Source: CAD feature listing. Evaluate the final solid. Frame: model axes, mm. Face numbers are marked on the shaded views. A direction names the side the tool comes from. Give positions to 0.01 mm unless a question says otherwise; leave off trailing zeros. Order: outer loops, then holes, each group sorted by start corner. A loop starts at its lowest first (then second) coordinate and runs counter-clockwise, first axis right, second up.
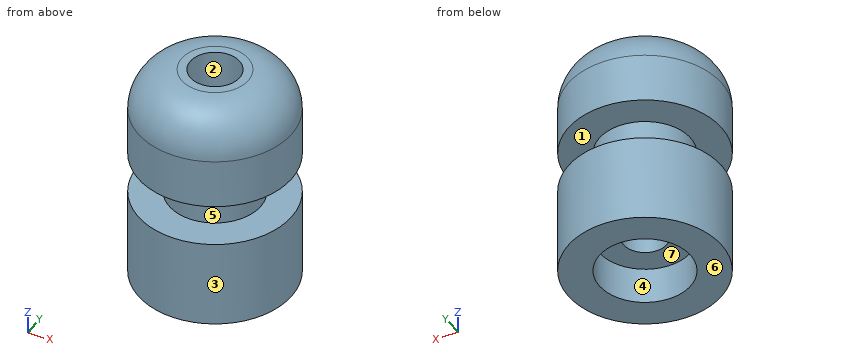
from build123d import *

# Parameters (mm, degrees)
F3_D = 10
F4_R = 10


with BuildPart() as f1:
    # F0 (on Front) → F1 (revolve)
    with BuildSketch(Plane.XZ):
        Polygon((7.1379574947, 42.9636351764), (-4.8425933346, 42.9636351764), (-4.8425933346, 27.8560947627), (-10.5409119278, 27.8560947627), (-10.5409119278, 0), (0, 0), (0, -8.4736431018), (7.1379574947, -8.4736431018), (7.1379574947, 11.8357595056), (0, 11.8357595056), (0, 21.5210486203), (7.1379574947, 21.5210486203), align=None)
    revolve(axis=Axis((-10.5409119278, 0, 16.1306988448), (0, 0, -1)))

    # F3 (through all)
    with Locations(Plane(origin=(0, 0, 0), x_dir=(1, 0, 0), z_dir=(0, 0, -1))):
        with Locations((-10.5409119278, 0)):
            Hole(F3_D / 2)

    # F4
    f4_edges = [f1.edges().sort_by_distance(p)[0] for p in [
        (-28.219781, 0, 42.963635),
    ]]
    fillet(f4_edges, radius=F4_R)


solid = f1.part
1) Section query A-A on z = -3. Output: boundary loops of the cut face in (x, y), and give its area (3 significant figures).
Checks:
outline: circle Ø35.36 at (-10.54, 0); hole circle Ø21.08 at (-10.54, 0)
area: 633 mm2
2) Ray query, L1, parallel to X at y = 0, z = -3.5; L2, parallel to Z at x = -15, y = -11; L3, parallel to Z at x = 5, y = -4. Return the intervals inside material, ascending.
Checks:
L1: x = -28.22 to -21.08, 0 to 7.14
L2: z = -8.47 to 11.84, 21.52 to 42.04
L3: z = -8.47 to 11.84, 21.52 to 38.44
3) Section query B-B on z = 10.5. Output: boundary loops of the cut face in (x, y).
Checks:
outline: circle Ø35.36 at (-10.54, 0); hole circle Ø10 at (-10.54, 0)
4) Pull-direction query (X, two-part tool) for the marked faces 4, 5, 6 and 7; classes: +X half, -X half, draft (parallel to the pull), parting line (faces both ways), or undercut.
Checks:
face 4: undercut
face 5: parting line
face 6: draft
face 7: undercut
5) First-contact query: pin 1 Ø3 at (x, z) = (-15.5, 13) entering from +Y; pin 2 Ø4 at (x, z) = (-14.5, 9.5) entering from +Y; pin 3 Ø10 at (x, y) = (-7.5, -4) entering from +Z; pin 4 Ø1.5 at (x, y) = (-17, 6) entering from -Z. Flat tips, straight axial feed; report the tip coordinate or a pass-through.
Checks:
pin 1: stops at y = 17.22
pin 2: stops at y = 17.57
pin 3: stops at z = 42.96
pin 4: stops at z = 0
6) Reachability of the marked faces 1, 2 and 3 from +Z, -Z, +X, -X, +Y, -Y: full face, straight path, thin tool, end or side. Return the list, or none.
Checks:
face 1: none
face 2: +Z
face 3: +Z, -Z
